```python
from build123d import *

# Parameters (mm, degrees)
F1_ANGLE_BACK = 45
F1_ANGLE      = 90


# Not quite as in the source:
# - ends of sketch curves that miss each other by under 0.0002 mm in the source are joined


with BuildPart() as f1:
    # F0 (on Front) → F1 (revolve)
    with BuildSketch(Plane.XZ, mode=Mode.PRIVATE) as f1_sk:
        Polygon((8, 4.2551231384), (8, 0), (9, 0), (9, 8.5), (8, 8.5), (8, 6.2273216248), align=None)
        Polygon((1, 2.124959883), (1, 4.2499679064), (1, 8.5), (0, 8.5), (0, 0), (1, 0), align=None)
        with BuildLine():
            add(Edge.make_bspline(
                [(1.6135353927, 4.7835650405), (1.6750901529, 4.970267715), (1.9288235062, 5.5585034544), (2.3534665623, 5.9191497273), (2.7, 5.9499679064)],
                knots=[0.2683438661, 0.2683438661, 0.2683438661, 0.2683438661, 0.5126436151, 1, 1, 1, 1], degree=3))
            Line((2.7, 5.9499679064), (2.7, 6.4499679064))
            add(Edge.make_bspline(
                [(1, 4.2499679064), (1.0015353048, 4.5626104683), (1.4551687546, 5.9442127178), (2.3433097433, 6.4271380926), (2.7, 6.4499679064)],
                knots=[0, 0, 0, 0, 0.5304369026, 1, 1, 1, 1], degree=3))
            Line((1, 4.2499679064), (1.4618344062, 4.2499679064))
            Line((1.4618344062, 4.2499679064), (1.5469024263, 4.5491884505))
            add(Edge.make_bspline(
                [(1.5469024263, 4.5491884505), (1.5645406816, 4.6235882391), (1.5868631876, 4.702665172), (1.6135353927, 4.7835650405)],
                knots=[0.1624866916, 0.1624866916, 0.1624866916, 0.1624866916, 0.2683438661, 0.2683438661, 0.2683438661, 0.2683438661], degree=3))
        make_face()
        with BuildLine():
            add(Edge.make_bspline(
                [(8, 4.2551231384), (7.9986488935, 3.9799898766), (7.7456702226, 2.8557466438), (6.505031952, 2.0758276235), (6.1, 2.0499037191)],
                knots=[0, 0, 0, 0, 0.4667977205, 1, 1, 1, 1], degree=3))
            Line((8, 4.2551231384), (8, 6.2273216248))
            Line((8, 6.2273216248), (7.9344944983, 5.4252070189))
            Line((7.9344944983, 5.4252070189), (7.801741117, 4.7100675088))
            Line((7.801741117, 4.7100675088), (7.6594823926, 4.2259131372))
            Line((7.6594823926, 4.2259131372), (7.5023478676, 3.7956271327))
            add(Edge.make_bspline(
                [(7.5023478676, 3.7956271327), (7.4950709382, 3.7744309229), (7.487268414, 3.753028112), (7.4789151485, 3.7314606417)],
                knots=[0.2362923479, 0.2362923479, 0.2362923479, 0.2362923479, 0.2672769863, 0.2672769863, 0.2672769863, 0.2672769863], degree=3))
            add(Edge.make_bspline(
                [(7.4789151485, 3.7314606417), (7.429977914, 3.6051085751), (7.1561404277, 3.07227024), (6.4919298971, 2.5847591313), (6.1, 2.5499037191)],
                knots=[0.2672769863, 0.2672769863, 0.2672769863, 0.2672769863, 0.4487991142, 1, 1, 1, 1], degree=3))
            add(Edge.make_bspline(
                [(6.1, 2.5499037191), (5.722922109, 2.560753403), (4.9562868612, 3.0652346955), (4.6679732537, 3.9028036589), (4.6499999995, 4.249903719)],
                knots=[0, 0, 0, 0, 0.5008610447, 1, 1, 1, 1], degree=3))
            add(Edge.make_bspline(
                [(2.7, 6.4499679064), (3.0971914861, 6.4159367347), (4.0379566942, 6.1199675516), (4.6572574431, 4.6342403799), (4.6499999995, 4.249903719)],
                knots=[0, 0, 0, 0, 0.4611151657, 0.9982015649, 0.9982015649, 0.9982015649, 0.9982015649], degree=3))
            Line((2.7, 6.4499679064), (2.7, 5.9499679064))
            add(Edge.make_bspline(
                [(2.7, 5.9499679064), (3.0770804596, 5.9391181486), (3.8437046032, 5.4345511486), (4.1320268683, 4.5970014065), (4.1499999995, 4.249903719)],
                knots=[0, 0, 0, 0, 0.5008644565, 1, 1, 1, 1], degree=3))
            add(Edge.make_bspline(
                [(4.3999999995, 3.3776864381), (4.2426068049, 3.7097412493), (4.1460321192, 4.0410870495), (4.1499999995, 4.249903719)],
                knots=[0.7063927669, 0.7063927669, 0.7063927669, 0.7063927669, 0.9982015652, 0.9982015652, 0.9982015652, 0.9982015652], degree=3))
            add(Edge.make_bspline(
                [(6.1, 2.0499037191), (5.7028107176, 2.0839347019), (5.0370554507, 2.2933169546), (4.5322969972, 3.0985774544), (4.3999999995, 3.3776864381)],
                knots=[0, 0, 0, 0, 0.4611126073, 0.7063927669, 0.7063927669, 0.7063927669, 0.7063927669], degree=3))
        make_face()
        with BuildLine():
            Line((1.5469024263, 4.5491884505), (1.6135353927, 4.7835650405))
            add(Edge.make_bspline(
                [(1.5469024263, 4.5491884505), (1.5645406816, 4.6235882391), (1.5868631876, 4.702665172), (1.6135353927, 4.7835650405)],
                knots=[0.1624866916, 0.1624866916, 0.1624866916, 0.1624866916, 0.2683438661, 0.2683438661, 0.2683438661, 0.2683438661], degree=3))
        make_face()
        Polygon((1.4618344062, 4.2499679064), (1, 4.2499679064), (1, 2.124959883), (1.0774135864, 2.6683010762), (1.144714681, 3.0744322246), (1.2561492896, 3.5201706593), (1.3731569326, 3.9380513733), align=None)
        with BuildLine():
            add(Edge.make_bspline(
                [(1.5, 4.2499679064), (1.5037909347, 4.3318066745), (1.5198283827, 4.4349876364), (1.5469024263, 4.5491884505)],
                knots=[0, 0, 0, 0, 0.1624866916, 0.1624866916, 0.1624866916, 0.1624866916], degree=3))
            Line((1.5469024263, 4.5491884505), (1.4618344062, 4.2499679064))
            Line((1.4618344062, 4.2499679064), (1.5, 4.2499679064))
        make_face()
    revolve(f1_sk.sketch.rotate(Axis((-22.7, 0, 2.7579944581), (0, 0, 1)), -F1_ANGLE_BACK), axis=Axis((-22.7, 0, 2.7579944581), (0, 0, 1)), revolution_arc=F1_ANGLE)


solid = f1.part
```
The model under review builds one solid part; all positions refer to its coordinate system, in mm. A direction names the side the tool comes from. Give positions to 0.01 mm unless a question says otherwise; leave off trailing zeros. Loops run counter-clockwise (first coordinate to the right, second up) from the corner with the lowest first, then second, coordinate; pieces in that order, holes last. Notation, with made-up numbers: (16.25, 3.25) - (42.25, 3.25) arc R22 cw to (42.25, 21.25) - close; hole circle Ø4 at (-40, 13.5). An arc over 180 degrees is marked (long way). Answer as a JSON object with one key per item and string values.
Q1. For faces 4 (the conical face through (1.103, -0.262, 2.829)), 5 (the flat face through (-3.5, -19.2, 4.3)), 6 (the cylindrical face through (8, 0, 7)), list the 3-axis set-ups (+Z, -Z, +X, -X, +Y, -Y) from which the entire face can be reached by the end or side of a thin tool; tool diameter is ignored.
Worked out:
{"face 4": "-Z", "face 5": "+Z, -Z, -X, -Y", "face 6": "+Z"}
Q2. Add section A-A on z = 7. State the section outline as (x, y) points, plus the area to 3 significant figures.
Worked out:
{"outline": "(-6.65, -16.05) - (-5.94, -16.76) arc R23.7 ccw to (-5.94, 16.76) - (-6.65, 16.05) arc R22.7 cw to start; (-0.99, -21.71) - (-0.28, -22.42) arc R31.7 ccw to (-0.28, 22.42) - (-0.99, 21.71) arc R30.7 cw to start", "area": "85.5 mm^2"}
Q3. Insertion check: pin 1 (1.5 mm diameter, centred on x = 3.5, z = 4, fed in from -Y); pin 2 (5 mm diameter, centred on y = 13, z = 6.5, fed in from +X); pin 3 (1.5 mm diameter, centred on x = 1, z = 4, fed in from +Y). Each pin has a flat end and moves straight along its axis. Give the tip position at first contact, or say it passes through.
Worked out:
{"pin 1": "stops at y = -18.9", "pin 2": "stops at x = 7.21", "pin 3": "stops at y = 21.87"}
Q4. Mouldability with a two-part tool opening along Y and no side actions: class faces 1 (the flat face through (0.3, 0, 0)), 2 (the flat face through (-3.5, 19.2, 4.3)), 3 (the conical face through (1.2, -0.3, 3.3)) as +Y half, -Y half, draft (parallel to the pull), parting line (faces both ways), or undercut.
Worked out:
{"face 1": "draft", "face 2": "+Y half", "face 3": "undercut"}
Q5. To check wall thickness, follow line 1 along X through (y, z) = (16, 3.5); line 2 along Y through (x, z) = (5.25, 3.75); line 3 along X through (y, z) = (16.5, 3.25). State the ranges of each line that lie inside material, in increasing order.
Worked out:
{"line 1": "x = -6.6 to -4.88, -0.9 to -0.27, 2.76 to 3.3, 3.5 to 4.67", "line 2": "y = -14.96 to -12.7, -12.49 to -11.4, 11.4 to 12.49, 12.7 to 14.96", "line 3": "x = -6.2 to -5.43, -1.12 to -0.45, 2.23 to 2.84, 3.19 to 4.37"}
